from build123d import *

# Parameters (mm, degrees)
SKETCH_1_W      = 20
SKETCH_1_H      = 20
EXTRUDE_1_DEPTH = 10
SKETCH_2_R      = 5
EXTRUDE_2_DEPTH = 10


with BuildPart() as part:
    # 草图1 → 凸台-拉伸1 (new, symmetric)
    with BuildSketch(Plane.XY):
        Rectangle(SKETCH_1_W, SKETCH_1_H)
    extrude(amount=EXTRUDE_1_DEPTH, both=True)

    # 草图2 → 凸台-拉伸2 (add)
    with BuildSketch(Plane(origin=(10, 0, 0), x_dir=(0, 0, -1), z_dir=(1, 0, 0))):
        Circle(SKETCH_2_R)
    extrude(amount=EXTRUDE_2_DEPTH)


solid = part.part
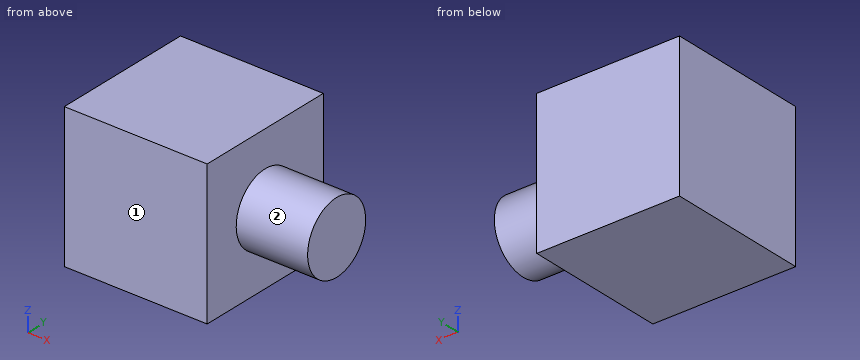
The listing builds one solid part. Answer for the finished solid, in the listing's coordinates (mm). Face numbers are marked on the shaded views. A direction names the side the tool comes from. Give positions to 0.01 mm unless a question says otherwise; leave off trailing zeros. Write each loop counter-clockwise with the first axis right and the second up, starting at its lowest first coordinate (ties: lowest second). Pieces come first, ordered by that corner, then holes. Notation, with made-up numbers: (20, 11) - (52, 11) arc R27 cw to (52, 44) - close; hole circle Ø2 at (49.5, -23). An arc over 180 degrees is marked (long way). Use a Markdown table: item, result.
1. This flat-tipped pin is pushed along its axis until it touches: P1, Ø4, axis at x = 16, y = -1.5, coming from the -Z side. Where does it stop, or does it pass through?
Values follow:
| item | result |
|---|---|
| P1 | stops at z = -5 |
2. A tool of negligible diameter and unlimited length cuts with its end or side. For the marked faces 1 and 2, from which of +Z, -Z, +X, -X, +Y, -Y can it reach the whole face along a straight path? Write none if from no direction.
Values follow:
| item | result |
|---|---|
| face 1 | +Z, -Z, +X, -X, -Y |
| face 2 | +X |
3. Section B-B on z = -3 is taken. Write down the section's boundary in (x, y).
Values follow:
| item | result |
|---|---|
| outline | (-10, -10) - (10, -10) - (10, -4) - (20, -4) - (20, 4) - (10, 4) - (10, 10) - (-10, 10) - close |
4. Find the intervals of material crossed by probe 1 along X at (y, z) = (8.5, -1); probe 2 along Z at (x, y) = (11.25, -0.5); probe 3 along Y at (x, z) = (11, -1), in increasing order. Write a range as from..to.
Values follow:
| item | result |
|---|---|
| probe 1 | x = -10..10 |
| probe 2 | z = -4.97..4.97 |
| probe 3 | y = -4.9..4.9 |
5. Section C-C on y = 6.75 is taken. Write down the section's boundary in (x, z), plus the area to 3 significant figures.
Values follow:
| item | result |
|---|---|
| outline | (-10, -10) - (10, -10) - (10, 10) - (-10, 10) - close |
| area | 400 mm² |
6. Section A-A on y = -4 is taken. Write down the section's boundary in (x, z).
Values follow:
| item | result |
|---|---|
| outline | (-10, -10) - (10, -10) - (10, -3) - (20, -3) - (20, 3) - (10, 3) - (10, 10) - (-10, 10) - close |
